The model under review builds one solid part; all positions refer to its coordinate system, in mm. Face numbers are marked on the shaded views. A direction names the side the tool comes from. Round coordinates to 2 decimals unless told otherwise and drop trailing zeros. Loops run counter-clockwise (first coordinate to the right, second up) from the corner with the lowest first, then second, coordinate; pieces in that order, holes last. Notation, with made-up numbers: (-9.75, 20.25) -> (27.25, 20.25) arc R9 ccw to (27.25, 27.25) -> close; hole circle Ø2 at (-2, 23). An arc over 180 degrees is marked (long way). Use a Markdown table: item, result. Add a question column.
1) Consider section C-C on z = -57. Give the boundary of the cut face in (x, y) (3 decimals).
2) Consider section A-A on x = -2. Give the boundary of the cut face in (y, z) (3 decimals).
3) For the marked faces 5 and 6, list the 3-axis set-ups (+Z, -Z, +X, -X, +Y, -Y) from which the entire face can be reached by the end or side of a thin tool; tool diameter is ignored.
4) Wall thickness on probe 1 along X at (y, z) = (-1, 29) (3 decimals): over which ranges is the line inside the solid? List them lowest first.
5) Mouldability with a two-part tool opening along X and no side actions: class the marked faces 1, 2, 3 and 4 as released by +X, released by -X, zero draft, split by the parting line, or undercut.
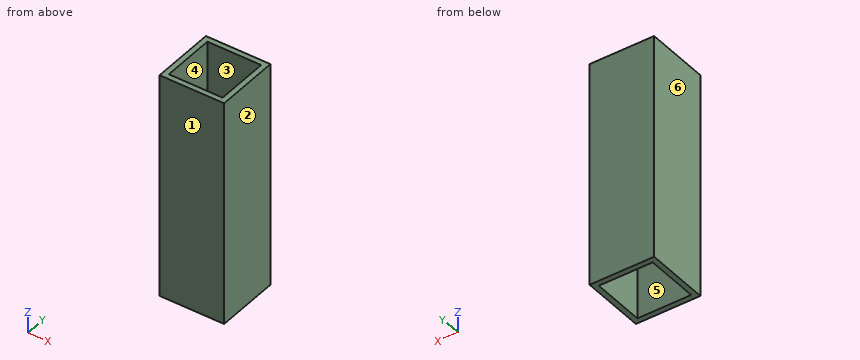
from build123d import *

# Parameters (mm, degrees)
SKETCH1_W           = 38.1
SKETCH1_H           = 133.35
BOSS_EXTRUDE1_DEPTH = 19.05
SKETCH2_W           = 31.75
SKETCH2_H           = 31.75
CUT_EXTRUDE1_DEPTH  = 134.35


with BuildPart() as part:
    # Sketch1 → Boss-Extrude1 (new body, symmetric)
    with BuildSketch(Plane(origin=(0, 0, 0), x_dir=(1, 0, 0), z_dir=(0, 1, 0))):
        Rectangle(SKETCH1_W, SKETCH1_H)
    extrude(amount=BOSS_EXTRUDE1_DEPTH, both=True)

    # Sketch2 → Cut-Extrude1 (cut, through all)
    with BuildSketch(Plane.XY.offset(66.675)):
        Rectangle(SKETCH2_W, SKETCH2_H)
    extrude(amount=-CUT_EXTRUDE1_DEPTH, mode=Mode.SUBTRACT)


solid = part.part
Result set:
| question | item | result |
|---|---|---|
| 1 | outline | (-19.05, -19.05) -> (19.05, -19.05) -> (19.05, 19.05) -> (-19.05, 19.05) -> close; hole (-15.875, -15.875) -> (15.875, -15.875) -> (15.875, 15.875) -> (-15.875, 15.875) -> close |
| 2 | outline | (-19.05, -66.675) -> (-15.875, -66.675) -> (-15.875, 66.675) -> (-19.05, 66.675) -> close; (15.875, -66.675) -> (19.05, -66.675) -> (19.05, 66.675) -> (15.875, 66.675) -> close |
| 3 | face 5 | +Z, -Z |
| 3 | face 6 | +Z, -Z, -X, +Y, -Y |
| 4 | probe 1 | -19.05 to -15.875, 15.875 to 19.05 |
| 5 | face 1 | zero draft |
| 5 | face 2 | released by +X |
| 5 | face 3 | undercut |
| 5 | face 4 | undercut |
